For this review, use the dimensioned drawing (mm, ordinates from the lowest corner) and the shaded views. Round coordinates to 2 decimals unless told otherwise and drop trailing zeros. Order: outer loops, then holes, each group sorted by start corner. A loop starts at its lowest first (then second) coordinate and runs counter-clockwise, first axis right, second up. Notation, with made-up numbers: M 13.5,77 L 24.5,77 A14 cw 24.5,94 Z; hole C 77.5,82 d1. An arc over 180 degrees is marked long. Answer as CSV lines item,"result". Start each with the question number.
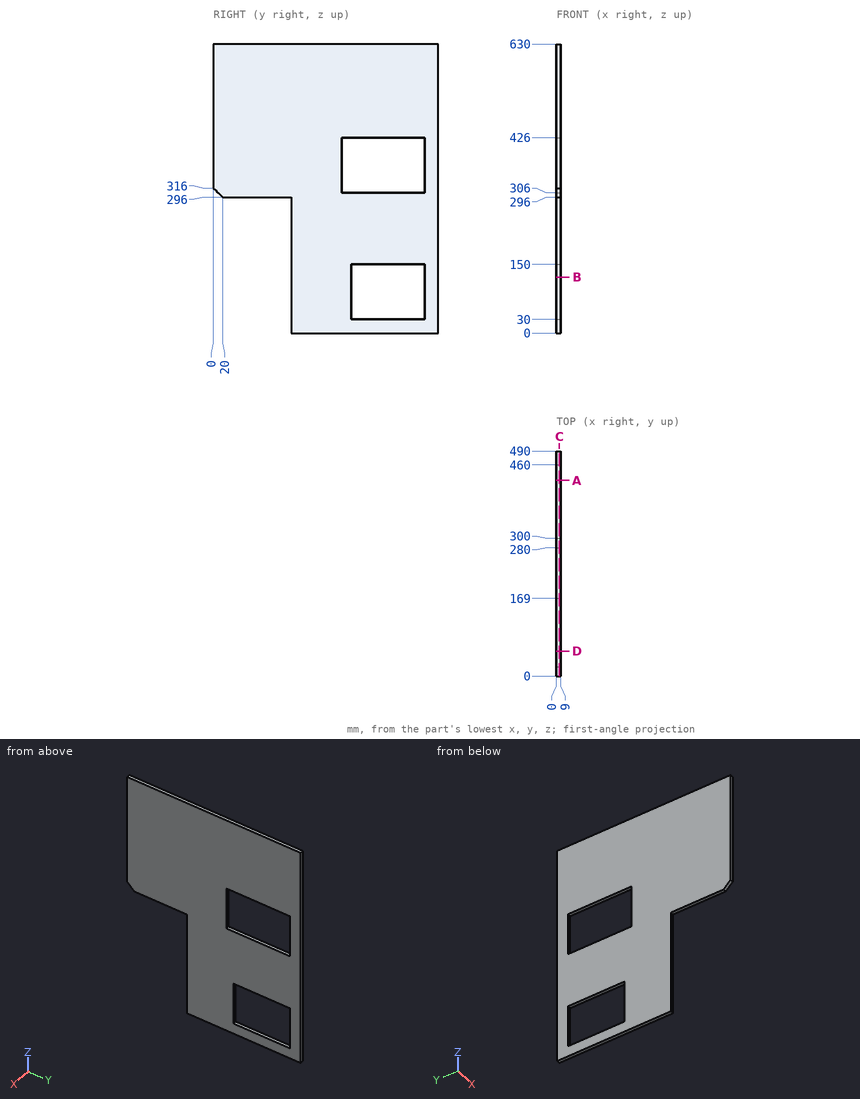
Item 1: Consider section A-A (y = 426). State the section outline as (x, z) points, and give its area (3 significant figures).
Item 2: Consider section B-B (z = 122). State the section outline as (x, y) points, and give its area (3 significant figures).
Item 3: Consider section C-C (x = 6.5). State the section outline as (y, z) points, and give its area (3 significant figures).
Item 4: Wall thickness on probe 1 along Z at (x, y) = (7.25, 364.5); probe 2 along Y at (x, z) = (3.5, 114.5); probe 3 along Y at (x, z) = (1.5, 385.5): over which ranges is each line inside the solid? List them lowest first. Write a range as [from, to].
Item 5: For pin 1 (4.5 mm diameter, centred on x = 4, z = 105, fed in from -Y); pin 2 (2.5 mm diameter, centred on x = 3, y = 117.5, fed in from -Z), all flat-tipped, find the tip position at first contact; note any pin that passes through.
Item 6: Consider section D-D (y = 54). State the section outline as (x, z) points.
Reported:
1,outline,"M 0,0 L 9,0 L 9,30 L 0,30 Z; M 0,150 L 9,150 L 9,306 L 0,306 Z; M 0,426 L 9,426 L 9,630 L 0,630 Z"
1,area,"3,510 mm²"
2,outline,"M 0,169 L 9,169 L 9,300 L 0,300 Z; M 0,460 L 9,460 L 9,490 L 0,490 Z"
2,area,"1,450 mm²"
3,outline,"M 0,316 L 20,296 L 169,296 L 169,0 L 490,0 L 490,630 L 0,630 Z; hole M 280,306 L 460,306 L 460,426 L 280,426 Z; hole M 300,30 L 460,30 L 460,150 L 300,150 Z"
3,area,"218,000 mm²"
4,probe 1,"z = [0, 30], [150, 306], [426, 630]"
4,probe 2,"y = [169, 300], [460, 490]"
4,probe 3,"y = [0, 280], [460, 490]"
5,pin 1,"stops at y = 169"
5,pin 2,"stops at z = 296"
6,outline,"M 0,296 L 9,296 L 9,630 L 0,630 Z"
